Could you check a few things on this model? Use its own coordinates, in mm. Round coordinates to 2 decimals unless told otherwise and drop trailing zeros. Loops run counter-clockwise (first coordinate to the right, second up) from the corner with the lowest first, then second, coordinate; pieces in that order, holes last. Notation, with made-up numbers: (3, -36.75) -> (62, -36.75) arc R5 ccw to (62, -32.75) -> close; hole circle Ø3 at (65, -23.5). An arc over 180 degrees is marked (long way). One line per item, written item: value.
from build123d import *

# Parameters (mm, degrees)
BOSS_EXTRUDE1_DEPTH = 1
CHAMFER1_SIZE       = 0.5


with BuildPart() as part:
    # Sketch1 → Boss-Extrude1 (new body)
    with BuildSketch(Plane(origin=(0, 0, 0), x_dir=(1, 0, 0), z_dir=(0, 1, 0))):
        with BuildLine():
            Line((-11.325, 14.325), (11.325, 14.325))
            ThreePointArc((11.325, 14.325), (13.446320344, 13.446320344), (14.325, 11.325))
            Line((14.325, 11.325), (14.325, -11.325))
            ThreePointArc((14.325, -11.325), (13.446320344, -13.446320344), (11.325, -14.325))
            Line((11.325, -14.325), (-11.325, -14.325))
            ThreePointArc((-11.325, -14.325), (-13.446320344, -13.446320344), (-14.325, -11.325))
            Line((-14.325, -11.325), (-14.325, 11.325))
            ThreePointArc((-14.325, 11.325), (-13.446320344, 13.446320344), (-11.325, 14.325))
        make_face()
    extrude(amount=BOSS_EXTRUDE1_DEPTH)

    # Chamfer1
    chamfer1_edges = [part.edges().sort_by_distance(p)[0] for p in [
        (13.446320344, 1, 13.446320344),
        (14.325, 1, 0),
        (13.446320344, 1, -13.446320344),
        (0, 1, -14.325),
        (-13.446320344, 1, -13.446320344),
        (-14.325, 1, 0),
        (-13.446320344, 1, 13.446320344),
        (0, 1, 14.325),
    ]]
    chamfer(chamfer1_edges, length=CHAMFER1_SIZE)


solid = part.part
(1) I'm going to push a flat-ended pin straight in: pin 1 Ø4 at (x, z) = (-10.5, 9.5) entering from -Y. Where does the tip first touch, or does it pass through?
Recorded:
pin 1: y = 0
(2) If we section it at A-A, the plane y = 0.75: Please give me the cut outline in (x, z) (3 decimals).
Recorded:
outline: (-14.075, -11.325) arc R2.75 ccw to (-11.325, -14.075) -> (11.325, -14.075) arc R2.75 ccw to (14.075, -11.325) -> (14.075, 11.325) arc R2.75 ccw to (11.325, 14.075) -> (-11.325, 14.075) arc R2.75 ccw to (-14.075, 11.325) -> close
(3) If I drill on L1, parallel to Z at x = 6.25, y = 0.85 (3 decimals); L2, parallel to X at y = 0.95, z = 12.5; L3, parallel to Z at x = 13, y = 0.75, over which ranges is the centre line in solid material (lowest first)?
Recorded:
L1: -13.975 to 13.975
L2: -13.59 to 13.59
L3: -13.51 to 13.51
